Verification items for the finished model (mm, model axes). A direction names the side the tool comes from. Coordinates: 2 decimals unless noted, no trailing zeros. Loops run counter-clockwise (first coordinate to the right, second up) from the corner with the lowest first, then second, coordinate; pieces in that order, holes last.
Q1. Sectioned sample at D-D (x = 24). Enter the section's corners in (y, z).
Q2. Go/stop test with flat-tipped pins: P1, Ø6.5, axis at x = -11.5, z = -17, coming from the +Y side; P2, Ø10, axis at y = 3.5, z = -13, coming from the -X side; P3, Ø5, axis at x = -0.5, y = 14, coming from the +Z side; P4, Ø1, axis at y = 3.5, z = 11.5, coming from the -X side. Record where each tip stops, or that it passes through.
Q3. Sectioned sample at A-A (z = 0). Enter the section's corners in (x, y).
Q4. Material ranges on probe 1 along Y at (x, z) = (-8, -17); probe 2 along X at (y, z) = (-23.05, 0); probe 3 along Y at (x, z) = (1, -11.5), recorded low to high.
Q5. Sectioned sample at C-C (y = 2). Count the separate pieces of the cut face and the enclosed holes in it, then the cut area to 3 significant figures.
Q6. Access from +Z, -Z, +X, -X, +Y, -Y to the whole of each face (thin tool, end or side, straight path). Record for faces 1 (the face through (-14, -15, 18)), 2 (the face through (-4.88, -22.54, 1.08)).
```python
from build123d import *

# Parameters (mm, degrees)
STOCK_PART1_1_START       = -15
STOCK_PART1_1_OUTLINE_R   = 4
STOCK_PART1_1_DEPTH       = 30
STOCK_PART1_1_START_2     = -25
STOCK_PART1_1_2_OUTLINE_R = 27.5
STOCK_PART1_1_2_DEPTH     = 5
STOCK_PART1_1_START_3     = 20
STOCK_PART1_1_3_OUTLINE_R = 27.5
STOCK_PART1_1_3_DEPTH     = 5
STOCK_PART1_1_START_4     = -20
STOCK_PART1_1_4_OUTLINE_R = 2.5
STOCK_PART1_1_4_DEPTH     = 40
SKETCH1_R                 = 5
CUT_EXTRUDE1_DEPTH        = 10
SKETCH2_R                 = 5
BOSS_EXTRUDE1_DEPTH       = 10.4


# Read off the part's stored shape, not the designer's step: Stock-Part1-1
with BuildPart() as part:
    # Stock-Part1-1 outline → Stock-Part1-1 (new body)
    with BuildSketch(Plane(origin=(0, 0, 0), x_dir=(1, 0, 0), z_dir=(0, 1, 0)).offset(STOCK_PART1_1_START)):
        with Locations((-11.755705046, 16.180339887)):
            Circle(STOCK_PART1_1_OUTLINE_R)
        with Locations((0, 20)):
            Circle(STOCK_PART1_1_OUTLINE_R)
        with Locations((11.755705046, 16.180339887)):
            Circle(STOCK_PART1_1_OUTLINE_R)
        with Locations((19.021130326, 6.180339887)):
            Circle(STOCK_PART1_1_OUTLINE_R)
        with Locations((19.021130326, -6.180339887)):
            Circle(STOCK_PART1_1_OUTLINE_R)
        with Locations((11.755705046, -16.180339887)):
            Circle(STOCK_PART1_1_OUTLINE_R)
        with Locations((0, -20)):
            Circle(STOCK_PART1_1_OUTLINE_R)
        with Locations((-11.755705046, -16.180339887)):
            Circle(STOCK_PART1_1_OUTLINE_R)
        with Locations((-19.021130326, -6.180339887)):
            Circle(STOCK_PART1_1_OUTLINE_R)
        with Locations((-19.021130326, 6.180339887)):
            Circle(STOCK_PART1_1_OUTLINE_R)
    extrude(amount=STOCK_PART1_1_DEPTH)



with BuildPart() as body_2:
    # Stock-Part1-1 2 outline → Stock-Part1-1 2 (new body)
    with BuildSketch(Plane(origin=(0, 0, 0), x_dir=(1, 0, 0), z_dir=(0, 1, 0)).offset(STOCK_PART1_1_START_2)):
        Circle(STOCK_PART1_1_2_OUTLINE_R)
    extrude(amount=STOCK_PART1_1_2_DEPTH)


with BuildPart() as body_3:
    # Stock-Part1-1 3 outline → Stock-Part1-1 3 (new body)
    with BuildSketch(Plane(origin=(0, 0, 0), x_dir=(1, 0, 0), z_dir=(0, 1, 0)).offset(STOCK_PART1_1_START_3)):
        Circle(STOCK_PART1_1_3_OUTLINE_R)
    extrude(amount=STOCK_PART1_1_3_DEPTH)


with BuildPart() as part_1:
    add(part.part)

    add(body_2.part)  # Stock-Part1-1 4 merges body 2

    add(body_3.part)  # Stock-Part1-1 4 merges body 3
    # Stock-Part1-1 4 outline → Stock-Part1-1 4 (add)
    with BuildSketch(Plane(origin=(0, 0, 0), x_dir=(1, 0, 0), z_dir=(0, 1, 0)).offset(STOCK_PART1_1_START_4)):
        with Locations((-11.755705046, 16.180339887)):
            Circle(STOCK_PART1_1_4_OUTLINE_R)
        with Locations((0, 20)):
            Circle(STOCK_PART1_1_4_OUTLINE_R)
        with Locations((11.755705046, 16.180339888)):
            Circle(STOCK_PART1_1_4_OUTLINE_R)
        with Locations((19.021130326, 6.180339888)):
            Circle(STOCK_PART1_1_4_OUTLINE_R)
        with Locations((19.021130326, -6.180339887)):
            Circle(STOCK_PART1_1_4_OUTLINE_R)
        with Locations((11.755705046, -16.180339887)):
            Circle(STOCK_PART1_1_4_OUTLINE_R)
        with Locations((0, -20)):
            Circle(STOCK_PART1_1_4_OUTLINE_R)
        with Locations((-11.755705046, -16.180339888)):
            Circle(STOCK_PART1_1_4_OUTLINE_R)
        with Locations((-19.021130326, -6.180339888)):
            Circle(STOCK_PART1_1_4_OUTLINE_R)
        with Locations((-19.021130326, 6.180339887)):
            Circle(STOCK_PART1_1_4_OUTLINE_R)
    extrude(amount=STOCK_PART1_1_4_DEPTH)

    # Sketch1 → Cut-Extrude1 (cut)
    with BuildSketch(Plane.XZ.offset(25)):
        with Locations(Location((0, 0, 0), (0, 0, 270))):
            Circle(SKETCH1_R)
    extrude(amount=-CUT_EXTRUDE1_DEPTH, mode=Mode.SUBTRACT)

    # Sketch2 → Boss-Extrude1 (add)
    with BuildSketch(Plane(origin=(0, 25, 0), x_dir=(1, 0, 0), z_dir=(0, 1, 0))):
        with Locations(Location((0, 0, 0), (0, 0, 90))):
            Circle(SKETCH2_R)
    extrude(amount=BOSS_EXTRUDE1_DEPTH)


solid = part_1.part
```
Geometry check:
1. outline: (-25, -13.43) - (-20, -13.43) - (-20, 13.43) - (-25, 13.43) - close; (20, -13.43) - (25, -13.43) - (25, 13.43) - (20, 13.43) - close
2. P1: stops at y = 25
2. P2: stops at x = -22.58
2. P3: stops at z = 24
2. P4: passes through
3. outline: (-27.5, -25) - (-5, -25) - (-5, -20) - (-27.5, -20) - close; (-27.5, 20) - (27.5, 20) - (27.5, 25) - (5, 25) - (5, 35.4) - (-5, 35.4) - (-5, 25) - (-27.5, 25) - close; (5, -25) - (27.5, -25) - (27.5, -20) - (5, -20) - close
4. probe 1: y = -25 to -20, -15 to 15, 20 to 25
4. probe 2: x = -27.5 to -5, 5 to 27.5
4. probe 3: y = -25 to -20, 20 to 25
5. separate pieces: 10
5. enclosed holes: 0
5. area: 503 mm2
6. face 1: none
6. face 2: -Y
